Check sheet for the modelled part. Datum: model origin and axes. Units: mm. Face numbers are marked on the shaded views. A direction names the side the tool comes from. Round coordinates to 2 decimals unless told otherwise and drop trailing zeros. Order: outer loops, then holes, each group sorted by start corner. A loop starts at its lowest first (then second) coordinate and runs counter-clockwise, first axis right, second up.
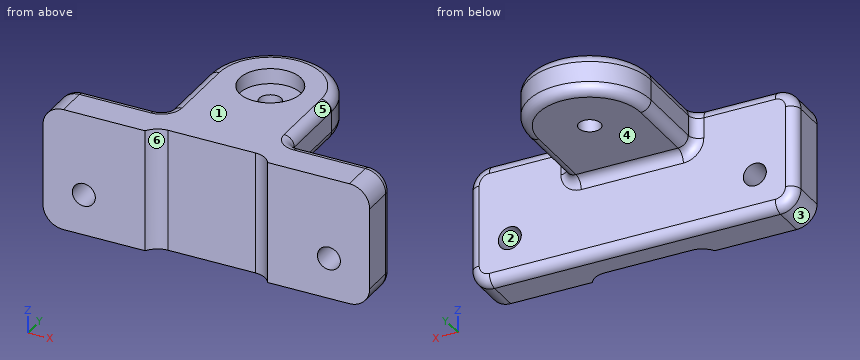
from build123d import *

# Parameters (mm, degrees)
SKETCH1_W                                = 101.6
SKETCH1_H                                = 38.1
BASE_EXTRUDE_DEPTH                       = 12.7
BOSS_EXTRUDE1_DEPTH                      = 12.7
CBORE_FOR_1_4_HEX_HEAD_BOLT1_D           = 6.7564
CBORE_FOR_1_4_HEX_HEAD_BOLT1_CBORE_D     = 19.05
CBORE_FOR_1_4_HEX_HEAD_BOLT1_CBORE_DEPTH = 4.7752
SKETCH10_W                               = 38.1
SKETCH10_H                               = 3.175
CUT_EXTRUDE1_DEPTH                       = 123.994494021
F_9_32_0_28125_DIAMETER_HOLE1_D          = 7.14375
FILLET1_R                                = 6.35
FILLET2_R                                = 3.175


with BuildPart() as part:
    # Sketch1 → Base-Extrude (new body)
    with BuildSketch(Plane(origin=(0, 0, 0), x_dir=(1, 0, 0), z_dir=(0, 1, 0))):
        with Locations((50.8, 19.05)):
            Rectangle(SKETCH1_W, SKETCH1_H)
    extrude(amount=BASE_EXTRUDE_DEPTH)

    # Sketch2 → Boss-Extrude1 (add)
    with BuildSketch(Plane.XY):
        with BuildLine():
            Line((31.75, 0), (31.75, 38.1))
            ThreePointArc((31.75, 38.1), (50.8, 57.15), (69.85, 38.1))
            Line((69.85, 38.1), (69.85, 0))
            Line((69.85, 0), (31.75, 0))
        make_face()
    extrude(amount=-BOSS_EXTRUDE1_DEPTH)

    # CBORE for 1/4 Hex Head Bolt1 (through all)
    with Locations(Plane(origin=(1.103556277, -5.640959644, 0), x_dir=(1, 0, 0), z_dir=(0, 0, 1))):
        with Locations((49.696443723, 43.740959644)):
            CounterBoreHole(CBORE_FOR_1_4_HEX_HEAD_BOLT1_D / 2, CBORE_FOR_1_4_HEX_HEAD_BOLT1_CBORE_D / 2, CBORE_FOR_1_4_HEX_HEAD_BOLT1_CBORE_DEPTH)

    # Sketch10 → Cut-Extrude1 (cut, through all)
    with BuildSketch(Plane(origin=(-1.071270925, 1.162093394, 0), x_dir=(1, 0, 0), z_dir=(0, 0, 1))):
        with Locations((51.871270925, 0.425406606)):
            Rectangle(SKETCH10_W, SKETCH10_H)
    extrude(amount=-CUT_EXTRUDE1_DEPTH, mode=Mode.SUBTRACT)

    # 9/32 (0.28125) Diameter Hole1 (through all)
    with Locations(Plane(origin=(45.908148148, 12.7, 7.855185185), x_dir=(-1, 0, 0), z_dir=(0, 1, 0))):
        with Locations((-42.991851852, -33.255185185), (33.208148148, -33.255185185)):
            Hole(F_9_32_0_28125_DIAMETER_HOLE1_D / 2)

    # Fillet1
    # the kernel refuses this fillet: 6.35 mm, written as the material it adds along each edge
    with BuildSketch(Plane(origin=(31.75, 3.175, 0), x_dir=(0, -1, 0), z_dir=(0, 0, -1))) as fillet1_piece_1:
        with BuildLine():
            CenterArc((6.35, -5.499261314), FILLET1_R, 120, 60)
            Line((0, -5.499261314), (0, 0))
            Line((0, 0), (3.175, 0))
        make_face()
    extrude(amount=38.1)
    with BuildSketch(Plane(origin=(69.85, 3.175, 0), x_dir=(-1, 0, 0), z_dir=(0, 0, -1))) as fillet1_piece_2:
        with BuildLine():
            CenterArc((5.499261314, -6.35), FILLET1_R, 90, 60)
            Line((0, -3.175), (0, 0))
            Line((0, 0), (5.499261314, 0))
        make_face()
    extrude(amount=38.1)
    # the kernel refuses this fillet: 6.35 mm, written as the material it takes off along each edge
    with BuildSketch(Plane(origin=(0, -15.875, -38.1), x_dir=(0, 0, 1), z_dir=(0, 1, 0)), Plane(origin=(0, -15.875, 0), x_dir=(1, 0, 0), z_dir=(0, 1, 0))) as fillet1_2_piece_1:
        with BuildLine():
            CenterArc((FILLET1_R, FILLET1_R), FILLET1_R, 180, 90)
            Line((0, FILLET1_R), (0, 0))
            Line((0, 0), (FILLET1_R, 0))
        make_face()
    extrude(amount=44.45, mode=Mode.SUBTRACT)
    with BuildSketch(Plane(origin=(101.6, -15.875, -38.1), x_dir=(0, 0, 1), z_dir=(0, 1, 0)), Plane(origin=(101.6, -15.875, 0), x_dir=(-1, 0, 0), z_dir=(0, 1, 0))) as fillet1_2_piece_2:
        with BuildLine():
            CenterArc((FILLET1_R, -FILLET1_R), FILLET1_R, 90, 90)
            Line((0, -FILLET1_R), (0, 0))
            Line((0, 0), (FILLET1_R, 0))
        make_face()
    extrude(amount=44.45, mode=Mode.SUBTRACT)

    # Fillet2
    fillet2_edges = [part.edges().sort_by_distance(p)[0] for p in [
        (82.55, 12.7, 0),
        (31.75, 25.4, -12.7),
        (69.85, 25.4, -12.7),
        (31.75, 25.4, 0),
        (69.85, 25.4, 0),
        (50.8, 57.15, 0),
        (31.75, 12.7, -6.35),
        (50.8, 57.15, -12.7),
        (69.85, 12.7, -6.35),
        (50.8, 12.7, -12.7),
        (19.05, 12.7, 0),
        (0, 12.7, -19.05),
        (101.6, 12.7, -19.05),
        (50.8, 12.7, -38.1),
        (1.859871939, 12.7, -36.240128061),
        (99.740128061, 12.7, -36.240128061),
        (99.740128061, 12.7, -1.859871939),
        (1.859871939, 12.7, -1.859871939),
    ]]
    fillet(fillet2_edges, radius=FILLET2_R)


solid = part.part
1) Sectioned sample at A-A on x = 50.8. Record the cut outline in (y, z) (3 decimals), and give its area (3 significant figures).
2) Sectioned sample at C-C on z = -23. Record the cut outline in (x, y) (3 decimals).
3) Sectioned sample at B-B on y = 4.5. Record the cut outline in (x, z), and give its area (3 significant figures).
4) Sectioned sample at D-D on x = 12.7. Record the cut outline in (y, z) (3 decimals), and give its area (3 significant figures).
5) Scan lines: line 1 (Z direction, x = 12.7, y = 6.25); line 2 (Y direction, x = 50.8, z = -2.8) (3 decimals); line 3 (Y direction, x = 50.8, z = -6.5) (3 decimals). Record each from-to range of solid material in increasing order.
6) Set-up check for the marked faces 4, 5 and 6: record each of +Z, -Z, +X, -X, +Y, -Y from which the full face is reachable in a straight line by a thin tool's end or side.
7) Gauge pin test, flat ends, axial feed: pin 1 (1.9 mm diameter, centred on y = 27.5, z = -7.5, fed in from +X); pin 2 (1 mm diameter, centred on x = 33.5, y = 41, fed in from +Z); pin 3 (12 mm diameter, centred on y = 25.5, z = -19, fed in from -X); pin 4 (9.5 mm diameter, centred on x = 47.5, z = -24.5, fed in from +Y). Record the tip position at first contact, or that the pin passes through.
8) Draft check along X on the marked faces 1, 2 and 3. Enter one of: pulls with the +X half, pulls with the -X half, needs draft (parallel to the pull), parting line crosses it, or undercut.
Values found:
1. outline: (3.175, -38.1) - (9.525, -38.1) arc R3.175 ccw to (12.7, -34.925) - (12.7, -15.875) arc R3.175 cw to (15.875, -12.7) - (34.722, -12.7) - (34.722, -4.775) - (28.575, -4.775) - (28.575, 0) - (3.175, 0) - close; (41.478, -12.7) - (53.975, -12.7) arc R3.175 ccw to (57.15, -9.525) - (57.15, -3.175) arc R3.175 ccw to (53.975, 0) - (47.625, 0) - (47.625, -4.775) - (41.478, -4.775) - close
1. area: 779 mm2
2. outline: (0, 0) - (10.055, 0) - (10.055, 12.7) - (3.175, 12.7) arc R3.175 ccw to (0, 9.525) - close; (15.345, 0) - (31.75, 0) arc R6.35 cw to (37.249, 3.175) - (64.351, 3.175) arc R6.35 cw to (69.85, 0) - (86.255, 0) - (86.255, 12.7) - (15.345, 12.7) - close; (91.545, 0) - (101.6, 0) - (101.6, 9.525) arc R3.175 ccw to (98.425, 12.7) - (91.545, 12.7) - close
3. outline: (0, -31.75) arc R6.35 ccw to (6.35, -38.1) - (95.25, -38.1) arc R6.35 ccw to (101.6, -31.75) - (101.6, -6.35) arc R6.35 ccw to (95.25, 0) - (6.35, 0) arc R6.35 ccw to (0, -6.35) - close; hole circle Ø7.14 at (12.7, -25.4); hole circle Ø7.14 at (88.9, -25.4)
3. area: 3,760 mm2
4. outline: (0, -38.1) - (9.525, -38.1) arc R3.175 ccw to (12.7, -34.925) - (12.7, -28.972) - (0, -28.972) - close; (0, -21.828) - (12.7, -21.828) - (12.7, -3.175) arc R3.175 ccw to (9.525, 0) - (0, 0) - close
4. area: 389 mm2
5. line 1: z = -38.1 to -28.97, -21.83 to 0
5. line 2: y = 3.175 to 28.575, 47.625 to 57.128
5. line 3: y = 3.175 to 34.722, 41.478 to 57.15
6. face 4: -Z, +X, -X, +Y
6. face 5: +Z, +X, +Y
6. face 6: +Z, -Z, -Y
7. pin 1: stops at x = 69.85
7. pin 2: stops at z = -0.22
7. pin 3: passes through
7. pin 4: stops at y = 12.7
8. face 1: needs draft
8. face 2: undercut
8. face 3: pulls with the -X half
